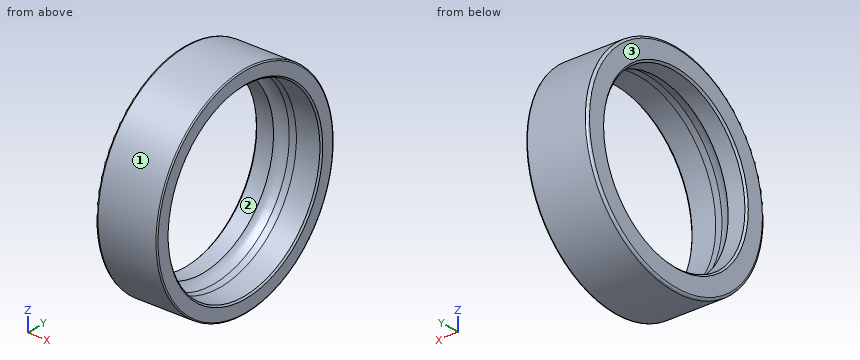
```python
from build123d import *


with BuildPart() as part:
    # Sketch1 → Revolve1 (revolve)
    with BuildSketch(Plane.XY, mode=Mode.PRIVATE) as revolve1_sk:
        with BuildLine():
            Line((-4, 11.465), (-3.76, 11.225))
            Line((-3.76, 11.225), (-1.567918365, 11.225))
            ThreePointArc((-1.567918365, 11.225), (-0.935852777, 11.758477094), (-0.141221865, 11.987968776))
            Line((-0.141221865, 11.987968776), (0.728253065, 12.05))
            Line((0.728253065, 12.05), (3.8, 12.05))
            Line((3.8, 12.05), (4, 12.25))
            Line((4, 12.25), (4, 13.85))
            ThreePointArc((4, 13.85), (3.956066017, 13.956066017), (3.85, 14))
            Line((3.85, 14), (-3.7, 14))
            ThreePointArc((-3.7, 14), (-3.912132034, 13.912132034), (-4, 13.7))
            Line((-4, 13.7), (-4, 11.465))
        make_face()
    revolve(revolve1_sk.sketch.rotate(Axis((4, 0, 0), (-1, 0, 0)), 270), axis=Axis((4, 0, 0), (-1, 0, 0)))


solid = part.part
```
Check sheet for the modelled part. Datum: model origin and axes. Units: mm. Face numbers are marked on the shaded views. Give positions to 0.01 mm unless a question says otherwise; leave off trailing zeros. Loops run counter-clockwise (first coordinate to the right, second up) from the corner with the lowest first, then second, coordinate; pieces in that order, holes last. Notation, with made-up numbers: M 48,59.5 L 69,59.5 A15 cw 69,76.5 Z; hole C 65.5,38 d7. An arc over 180 degrees is marked long. Answer in a Markdown table with one row per item.
1) Depth check by flat-ended pin: pin 1 (4 mm diameter, centred on x = -2.5, z = 6.5, fed in from -Y); pin 2 (1.5 mm diameter, centred on x = -1, y = 2, fed in from -Z); pin 3 (1.5 mm diameter, centred on x = 1.5, z = -9.5, fed in from +Y). Enter the tip coordinate at first touch or a pass-through.
Solutions:
| item | result |
|---|---|
| pin 1 | stops at y = -13.26 |
| pin 2 | stops at z = -13.94 |
| pin 3 | stops at y = 10.93 |
2) Cross-section at C-C (x = 2). Enter the section's corners in (y, z).
Solutions:
| item | result |
|---|---|
| outline | C 0,0 d28; hole C 0,0 d24.1 |
3) Mould release check, pull along Y, two halves, no side actions. Record for the marked faces 1, 2 and 3: released by +Y, released by -Y, zero draft, split by the parting line, or undercut.
Solutions:
| item | result |
|---|---|
| face 1 | split by the parting line |
| face 2 | undercut |
| face 3 | zero draft |
4) Cross-section at D-D (x = -2.25). Enter the section's corners in (y, z) (3 decimals).
Solutions:
| item | result |
|---|---|
| outline | C 0,0 d28; hole C 0,0 d22.45 |
5) Thickness scan on line 1 (Y direction, x = -2.6, z = 0) (3 decimals); line 2 (Y direction, x = 2.7, z = 0); line 3 (Z direction, x = 0, y = -1.25). Record the ranges inside material, lowest first.
Solutions:
| item | result |
|---|---|
| line 1 | y = -14 to -11.225, 11.225 to 14 |
| line 2 | y = -14 to -12.05, 12.05 to 14 |
| line 3 | z = -13.94 to -11.93, 11.93 to 13.94 |
